from build123d import *

# Parameters (mm, degrees)
BOSS_EXTRUDE1_DEPTH = 6.35
SKETCH2_W           = 12.7
SKETCH2_H           = 6.35
BOSS_EXTRUDE3_DEPTH = 32.9438
FILLET1_R           = 2.54
SKETCH3_W           = 17.78
SKETCH3_H           = 19.05
SKETCH3_R           = 2.0955
BOSS_EXTRUDE4_DEPTH = 6.35
FILLET2_R           = 3.81


with BuildPart() as part:
    # Sketch1 → Boss-Extrude1 (new body)
    with BuildSketch(Plane.XY):
        with BuildLine():
            Line((0, 0), (0, 69.85))
            Line((0, 69.85), (-12.7, 69.85))
            Line((-12.7, 69.85), (-19.325374009, 61.568282488))
            ThreePointArc((-19.325374009, 61.568282488), (-16.341038142, 54.373230514), (-24.015699161, 55.705376048))
            Line((-24.015699161, 55.705376048), (-31.75, 46.0375))
            Line((-31.75, 46.0375), (-50.8, 46.0375))
            Line((-50.8, 46.0375), (-50.8, 52.705))
            ThreePointArc((-50.8, 52.705), (-55.245, 57.15), (-50.8, 61.595))
            Line((-50.8, 61.595), (-50.8, 69.85))
            Line((-50.8, 69.85), (-63.5, 69.85))
            Line((-63.5, 69.85), (-63.5, 33.3375))
            Line((-63.5, 33.3375), (-12.7, 33.3375))
            Line((-12.7, 33.3375), (-12.7, 0))
            Line((-12.7, 0), (0, 0))
        make_face()
    extrude(amount=BOSS_EXTRUDE1_DEPTH)

    # Sketch2 → Boss-Extrude3 (add)
    with BuildSketch(Plane(origin=(0, 0, 6.35), x_dir=(-1, 0, 0), z_dir=(0, 0, -1))):
        with Locations((6.35, 66.675)):
            Rectangle(SKETCH2_W, SKETCH2_H)
        with Locations((57.15, 66.675)):
            Rectangle(SKETCH2_W, SKETCH2_H)
    extrude(amount=BOSS_EXTRUDE3_DEPTH)

    # Fillet1
    fillet1_edges = [part.edges().sort_by_distance(p)[0] for p in [
        (-57.15, 63.5, 0),
        (-6.35, 63.5, 0),
        (-12.7, 66.675, 0),
    ]]
    fillet(fillet1_edges, radius=FILLET1_R)

    # Sketch3 → Boss-Extrude4 (add)
    with BuildSketch(Plane.XY.offset(6.35)):
        with Locations((8.89, 41.65092)):
            Rectangle(SKETCH3_W, SKETCH3_H)
        with Locations((8.89, 41.65092)):
            Circle(SKETCH3_R, mode=Mode.SUBTRACT)
    extrude(amount=-BOSS_EXTRUDE4_DEPTH)

    # Fillet2
    fillet2_edges = [part.edges().sort_by_distance(p)[0] for p in [
        (17.78, 32.12592, 3.175),
        (17.78, 51.17592, 3.175),
        (0, 51.17592, 3.175),
        (0, 32.12592, 3.175),
        (-12.7, 33.3375, 3.175),
        (-50.8, 46.0375, 3.175),
        (-31.75, 46.0375, 3.175),
    ]]
    fillet(fillet2_edges, radius=FILLET2_R)


solid = part.part
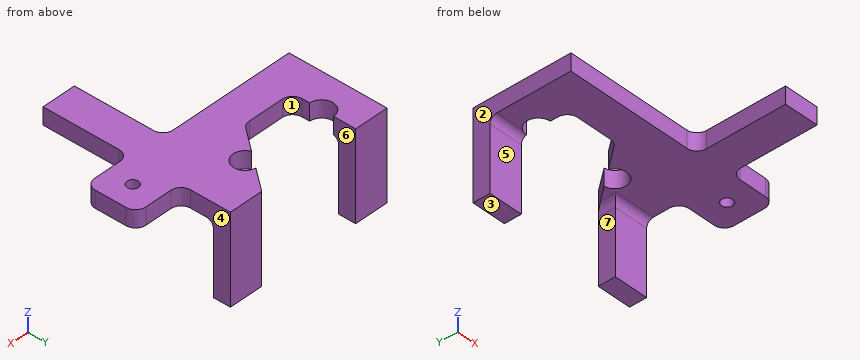
Geometry check sheet. Reference: the model listing, model coordinates, mm. Face numbers are marked on the shaded views. A direction names the side the tool comes from. Give positions to 0.01 mm unless a question says otherwise; leave off trailing zeros. Write each loop counter-clockwise with the first axis right and the second up, starting at its lowest first coordinate (ties: lowest second). Pieces come first, ordered by that corner, then holes. Notation, with made-up numbers: M 14,15 L 69,15 A22 ccw 69,49 Z; hole C 89.25,-12.5 d11. An arc over 180 degrees is marked long. One line per question, with ' | ' between items.
1. Cross-section at D-D (y = 18). Enter the section's corners in (x, z), plus the area to 3 significant figures.
Ans:
outline: M -12.7,0 L 0,0 L 0,6.35 L -12.7,6.35 Z | area: 80.6 mm2
2. Cross-section at A-A (z = -12). Enter the section's corners in (x, y), plus the area to 3 significant figures.
Ans:
outline: M -63.5,63.5 L -50.8,63.5 L -50.8,69.85 L -63.5,69.85 Z; M -12.7,63.5 L 0,63.5 L 0,69.85 L -12.7,69.85 Z | area: 161 mm2
3. Gauge pin test, flat ends, axial feed: pin 1 (10 mm diameter, centred on x = -56, z = -15.5, fed in from -Y); pin 2 (10 mm diameter, centred on y = 57, z = -2.5, fed in from +X); pin 3 (3 mm diameter, centred on y = 19.5, z = 4.5, fed in from -X); pin 4 (1 mm diameter, centred on x = 1, z = -11, fed in from +Y). Record the tip position at first contact, or that the pin passes through.
Ans:
pin 1: y = 63.5 | pin 2: x = 0.78 | pin 3: x = -12.7 | pin 4: through
4. Cross-section at B-B (y = 57.15). Enter the section's corners in (x, z) (3 decimals), plus the area to 3 significant figures.
Ans:
outline: M -63.5,0 L -55.245,0 L -55.245,6.35 L -63.5,6.35 Z; M -15.367,0 L 0,0 L 0,6.35 L -15.367,6.35 Z | area: 150 mm2
5. Set-up check for the marked faces 4, 5, 6 and 7: record each of +Z, -Z, +X, -X, +Y, -Y from which the full face is reachable in a straight line by a thin tool's end or side.
Ans:
face 4: +Z, -Z, +X, +Y | face 5: -Z, +X, -X, -Y | face 6: +Z, -Z, +Y | face 7: -Z, +Y, -Y
6. Mould release check, pull along X, two halves, no side actions. Record for the marked faces 1, 2 and 3: released by +X, released by -X, zero draft, split by the parting line, or undercut.
Ans:
face 1: undercut | face 2: released by -X | face 3: zero draft
7. Scan lines: line 1 along Y through (x, z) = (8.89, 3.25); line 2 along X through (y, z) = (57.15, 2.5) (3 decimals); line 3 along Y through (x, z) = (-9.5, -9). Record each from-to range of solid material in increasing order. Write a range as from..to.
Ans:
line 1: 32.13..39.56, 43.75..51.18 | line 2: -63.5..-55.245, -15.367..0 | line 3: 63.5..69.85
8. Cross-section at C-C (x = -4). Enter the section's corners in (y, z).
Ans:
outline: M 0,0 L 60.96,0 A2.54 cw 63.5,-2.54 L 63.5,-26.59 L 69.85,-26.59 L 69.85,6.35 L 0,6.35 Z
